The model under review builds one solid part; all positions refer to its coordinate system, in mm. A direction names the side the tool comes from. Round coordinates to 2 decimals unless told otherwise and drop trailing zeros. Loops run counter-clockwise (first coordinate to the right, second up) from the corner with the lowest first, then second, coordinate; pieces in that order, holes last. Notation, with made-up numbers: M -15.5,40.25 L 22.5,40.25 A6 cw 22.5,45.25 Z; hole C 81,50 d8. An arc over 180 degrees is marked long. Answer in a Markdown table with one row per item. Add a question column.
from build123d import *

# Parameters (mm, degrees)
F0_R      = 11.5
F1_DEPTH  = 10
F2_W      = 30.00446
F2_H      = 3
F3_DEPTH  = 3
F4_R      = 0.5
F5_DEPTH  = 1
F6_R      = 0.5
F7_DEPTH  = 1
F9_DEPTH  = 3
F11_DEPTH = 5


with BuildPart() as f1:
    # F0 (on Front) → F1 (new body)
    with BuildSketch(Plane.XZ):
        Circle(F0_R)
    extrude(amount=F1_DEPTH)

    # F2 (on face) → F3 (cut)
    with BuildSketch(Plane.XZ.offset(10)):
        Rectangle(F2_W, F2_H)
    extrude(amount=-F3_DEPTH, mode=Mode.SUBTRACT)

    # F4 (on face) → F5 (cut)
    with BuildSketch(Plane(origin=(0, 0, 1.5), x_dir=(1, 0, 0), z_dir=(0, 0, -1))):
        with Locations((-10.401754, 9)):
            Circle(F4_R)
    extrude(amount=-F5_DEPTH, mode=Mode.SUBTRACT)

    # F6 (on face) → F7 (cut)
    with BuildSketch(Plane.XY.offset(-1.5)):
        with Locations((-10.401754, -9)):
            Circle(F6_R)
    extrude(amount=-F7_DEPTH, mode=Mode.SUBTRACT)

    # F8 (on face) → F9 (cut)
    with BuildSketch(Plane.XY.offset(-1.5)):
        Polygon((13.954913, -2.917858), (3.598246, -7), (11.401754, -7), align=None)
        Polygon((14.351814, -7.2972), (13.954913, -2.917858), (11.401754, -7), align=None)
    extrude(amount=F9_DEPTH, mode=Mode.SUBTRACT)

    # F10 (on face) → F11 (cut)
    with BuildSketch(Plane(origin=(2.871931, -7.286281, 0), x_dir=(0.93034, 0.366699, 0), z_dir=(0.366699, -0.93034, 0))):
        with BuildLine():
            ThreePointArc((7.342269, -1.5), (8.402929, -1.06066), (8.842269, 0))
            ThreePointArc((8.842269, 0), (8.402929, 1.06066), (7.342269, 1.5))
            ThreePointArc((7.342269, 1.5), (5.842269, 0), (7.342269, -1.5))
        make_face()
        with BuildLine():
            ThreePointArc((7.342269, 1.5), (8.402929, 1.06066), (8.842269, 0))
            ThreePointArc((8.842269, 0), (8.402929, -1.06066), (7.342269, -1.5))
            Line((7.342269, -1.5), (11.188243, -1.5))
            Line((11.188243, -1.5), (11.188243, 1.5))
            Line((11.188243, 1.5), (7.342269, 1.5))
        make_face()
    extrude(amount=-F11_DEPTH, mode=Mode.SUBTRACT)


solid = f1.part
1. Take a section at D-D, the plane z = 0. State the section outline as (x, y) points.
2. Take a section at C-C, the plane y = -7.5. State the section outline as (x, z) points, and give its area (3 significant figures).
3. Take a section at B-B, the plane x = 0. State the section outline as (y, z) points.
4. For pin 1 Ø2 at (x, y) = (1, -7) entering from +Z; pin 2 Ø3 at (x, y) = (4, -3) entering from -Z (3 decimals), all flat-tipped, find the tip position at first contact; note any pin that passes through.
5. To check wall thickness, follow probe 1 along Z at (x, y) = (-7.75, -8.5); probe 2 along X at (y, z) = (-9, 2.25); probe 3 along Z at (x, y) = (0.5, -9.5). State the ranges of each line that lie inside material, in increasing order.
6. Machinability: for faces 5 (the flat face through (-4, -7, 0)), 6 (the flat face through (7.228, -0.195, 0.021)), 7 (the cylindrical face through (-10.51, -8.51, 1.99)), 8 (the flat face through (6.01, -6.05, -0.02)), which of the approach directions +Z, -Z, +X, -X, +Y, -Y give a long, thin tool a straight path to every point of the face, cutting with its end or side? Answer none if there is none.
7. Take a section at A-A, the plane y = -9. State the section outline as (x, z) points, and give its area (3 significant figures).
8. Mouldability with a two-part tool opening along Z and no side actions: class faces 1 (the flat face through (0, 0, 0)), 2 (the flat face through (-10.4, -9, -2.5)), 3 (the cylindrical face through (7.404, -2.851, 0.033)), 4 (the cylindrical face through (-11.49, -4.93, 0.48)) as released by +Z, released by -Z, zero draft, split by the parting line, or undercut.
Check sheet entries:
| question | item | result |
|---|---|---|
| 1 | outline | M -11.5,-7 L 3.6,-7 L 8.31,-5.14 L 6.47,-0.49 L 7.72,0 L -11.5,0 Z |
| 2 | outline | M -11.4,-1.5 A11.5 ccw 11.4,-1.5 Z; M -11.4,1.5 L 11.4,1.5 A11.5 ccw Z |
| 2 | area | 347 mm^2 |
| 3 | outline | M -10,-11.5 L 0,-11.5 L 0,11.5 L -10,11.5 L -10,1.5 L -7,1.5 L -7,-1.5 L -10,-1.5 Z |
| 4 | pin 1 | stops at z = 11.5 |
| 4 | pin 2 | stops at z = -11.225 |
| 5 | probe 1 | z = -8.5 to -1.5, 1.5 to 8.5 |
| 5 | probe 2 | x = -11.28 to -10.9, -9.9 to 11.28 |
| 5 | probe 3 | z = -11.49 to -1.5, 1.5 to 11.49 |
| 6 | face 5 | +X, -X, -Y |
| 6 | face 6 | +X |
| 6 | face 7 | none |
| 6 | face 8 | +X, -Y |
| 7 | outline | M -11.4,-1.5 A11.5 ccw 11.4,-1.5 L -9.9,-1.5 L -9.9,-2.5 L -10.9,-2.5 L -10.9,-1.5 Z; M -11.4,1.5 L -10.9,1.5 L -10.9,2.5 L -9.9,2.5 L -9.9,1.5 L 11.4,1.5 A11.5 ccw Z |
| 7 | area | 345 mm^2 |
| 8 | face 1 | zero draft |
| 8 | face 2 | undercut |
| 8 | face 3 | undercut |
| 8 | face 4 | split by the parting line |
